```python
from build123d import *

# Parameters (mm, degrees)
SKETCH_R       = 4.5
SKETCH_W       = 5
SKETCH_H       = 5
PAD_DEPTH      = 10
PAD_DEPTH_BACK = 25
SKETCH001_R    = 3
PAD001_DEPTH   = 1.5


with BuildPart() as part:
    # Sketch → Pad (new body, two sides)
    with BuildSketch(Plane.XY) as pad_sk:
        Circle(SKETCH_R)
        Rectangle(SKETCH_W, SKETCH_H, mode=Mode.SUBTRACT)
    extrude(amount=PAD_DEPTH)
    extrude(pad_sk.sketch, amount=-PAD_DEPTH_BACK)

    # Sketch001 → Pad001 (join, symmetric)
    with BuildSketch(Plane.XZ):
        with BuildLine():
            ThreePointArc((-8.258824, 20.364706), (-20.445693, 17.829727), (-13.5, 7.5))
            Line((-12, 7.5), (-13.5, 7.5))
            ThreePointArc((-4.5, 0), (-6.696699, 5.303301), (-12, 7.5))
            Line((-4.5, 0), (4.5, 0))
            ThreePointArc((12, 7.5), (6.696699, 5.303301), (4.5, 0))
            Line((12, 7.5), (13.5, 7.5))
            ThreePointArc((13.5, 7.5), (20.445693, 17.829727), (8.258824, 20.364706))
            ThreePointArc((-8.258824, 20.364706), (0, 17), (8.258824, 20.364706))
        make_face()
        with Locations((13.5, 15)):
            Circle(SKETCH001_R, mode=Mode.SUBTRACT)
        with Locations((-13.5, 15)):
            Circle(SKETCH001_R, mode=Mode.SUBTRACT)
    extrude(amount=PAD001_DEPTH, both=True)


solid = part.part
```
Model file for the job. Use its own axes, mm. A direction names the side the tool comes from. Give positions to 0.01 mm unless a question says otherwise; leave off trailing zeros. Loops run counter-clockwise (first coordinate to the right, second up) from the corner with the lowest first, then second, coordinate; pieces in that order, holes last. Notation, with made-up numbers: (61.25, -31) - (75.25, -31) arc R18 cw to (75.25, -12) - close; hole circle Ø7 at (-23.5, -19). An arc over 180 degrees is marked (long way). One line per item, written item: value. Start each with the question number.
1. Probe L1, parallel to Z at x = -13.5, y = 0.7; L2, parallel to X at y = -1, z = -0.5; L3, parallel to Z at x = 16, y = 0. List the from-to ranges inside material, lowest first. Write a range as from..to.
2. Slice it at A-A (z = 15). List the corners of the cut face in (x, y).
3. Which spindle directions (+Z, -Z, +X, -X, +Y, -Y) get a long thin tool onto all of the face, cutting with end or side? Do faces 4 (the flat face through (2.5, 0, -11)), 5 (the flat face through (13, 0, 7.5)), 6 (the flat face through (-13, 0, 7.5)). Say none if no direction does.
4. Pull direction Y, two halves, no side cores. Call faces 1 (the cylindrical face through (2.08, -3.99, -7.25)), 2 (the flat face through (-2.5, 0, -11)), 3 (the cylindrical face through (11.1, 0, 13.2)): pulls with the +Y half, pulls with the -Y half, needs draft (parallel to the pull), parting line crosses it, or undercut.
5. Slice it at D-D (x = -6.5). List the corners of the cut face in (y, z), plus the area to 3 significant figures.
6. Slice it at B-B (z = 4.5). List the corners of the cut face in (x, y).
7. Slice it at C-C (z = -9). List the corners of the cut face in (x, y), plus the area to 3 significant figures.
8. Pin check, flat tips, straight feed: pin 1 (1.2 mm diameter, centred on x = 12.5, y = -0.5, fed in from -Z); pin 2 (1.5 mm diameter, centred on x = -0.5, z = 1, fed in from -Y); pin 3 (1.5 mm diameter, centred on y = 0.5, z = -8, fed in from +X); pin 4 (8 mm diameter, centred on x = -9.5, z = 9.5, fed in from +Y). Stop position of each tip, or through.
Solution:
1. L1: z = 7.5..12, 18..22.5
1. L2: x = -4.39..-2.5, 2.5..4.39
1. L3: z = 7.93..13.34, 16.66..22.07
2. outline: (-21, -1.5) - (-16.5, -1.5) - (-16.5, 1.5) - (-21, 1.5) - close; (-10.5, -1.5) - (10.5, -1.5) - (10.5, 1.5) - (-10.5, 1.5) - close; (16.5, -1.5) - (21, -1.5) - (21, 1.5) - (16.5, 1.5) - close
3. face 4: -Z
3. face 5: -Z, +X, +Y, -Y
3. face 6: -Z, -X, +Y, -Y
4. face 1: parting line crosses it
4. face 2: undercut
4. face 3: needs draft
5. outline: (-1.5, 5.1) - (1.5, 5.1) - (1.5, 18.95) - (-1.5, 18.95) - close
5. area: 41.5 mm^2
6. outline: (-6, -1.5) - (-4.24, -1.5) arc R4.5 ccw to (4.24, -1.5) - (6, -1.5) - (6, 1.5) - (4.24, 1.5) arc R4.5 ccw to (-4.24, 1.5) - (-6, 1.5) - close; hole (-2.5, -2.5) - (2.5, -2.5) - (2.5, -1.5) - (-2.5, -1.5) - close; hole (-2.5, 1.5) - (2.5, 1.5) - (2.5, 2.5) - (-2.5, 2.5) - close
7. outline: circle Ø9 at (0, 0); hole (-2.5, -2.5) - (2.5, -2.5) - (2.5, 2.5) - (-2.5, 2.5) - close
7. area: 38.6 mm^2
8. pin 1: stops at z = 7.5
8. pin 2: stops at y = -4.5
8. pin 3: stops at x = 4.5
8. pin 4: stops at y = 1.5
